```python
from build123d import *
from OCP.BRepFilletAPI import BRepFilletAPI_MakeChamfer

# Parameters (mm, degrees)
SKETCH1_W           = 16
SKETCH1_H           = 16
BOSS_EXTRUDE1_DEPTH = 10
SKETCH2_R           = 4
CUT_EXTRUDE1_DEPTH  = 1
FILLET4_SIZE        = 2
FILLET4_SIZE2       = 1.2


with BuildPart() as part:
    # Sketch1 → Boss-Extrude1 (new body)
    with BuildSketch(Plane.XY):
        with Locations((8, 8)):
            Rectangle(SKETCH1_W, SKETCH1_H)
    extrude(amount=BOSS_EXTRUDE1_DEPTH)

    # Sketch2 → Cut-Extrude1 (cut)
    with BuildSketch(Plane.XY.offset(10)):
        with Locations((8, 8)):
            Circle(SKETCH2_R)
    extrude(amount=-CUT_EXTRUDE1_DEPTH, mode=Mode.SUBTRACT)

    # Fillet4: one chamfer whose edges measure the first distance from different faces: ONE call of the kernel's chamfer builder (chamfer() names one face for all edges)
    fillet4_edges_1 = [part.edges().sort_by_distance(p)[0] for p in [
        (16, 8, 10),
    ]]
    fillet4_side_1 = [part.faces().sort_by_distance(p)[0] for p in [
        (16, 8, 5),
    ]]
    fillet4_edges_2 = [part.edges().sort_by_distance(p)[0] for p in [
        (8, 16, 10),
    ]]
    fillet4_side_2 = [part.faces().sort_by_distance(p)[0] for p in [
        (8, 16, 5),
    ]]
    fillet4_edges_3 = [part.edges().sort_by_distance(p)[0] for p in [
        (0, 8, 10),
    ]]
    fillet4_side_3 = [part.faces().sort_by_distance(p)[0] for p in [
        (0, 8, 5),
    ]]
    fillet4_edges_4 = [part.edges().sort_by_distance(p)[0] for p in [
        (8, 0, 10),
    ]]
    fillet4_side_4 = [part.faces().sort_by_distance(p)[0] for p in [
        (8, 0, 5),
    ]]
    fillet4 = BRepFilletAPI_MakeChamfer(part.part.solid().wrapped)
    for e in fillet4_edges_1:
        fillet4.Add(FILLET4_SIZE, FILLET4_SIZE2, e.wrapped, fillet4_side_1[0].wrapped)  # the first distance lies on this face
    for e in fillet4_edges_2:
        fillet4.Add(FILLET4_SIZE, FILLET4_SIZE2, e.wrapped, fillet4_side_2[0].wrapped)  # the first distance lies on this face
    for e in fillet4_edges_3:
        fillet4.Add(FILLET4_SIZE, FILLET4_SIZE2, e.wrapped, fillet4_side_3[0].wrapped)  # the first distance lies on this face
    for e in fillet4_edges_4:
        fillet4.Add(FILLET4_SIZE, FILLET4_SIZE2, e.wrapped, fillet4_side_4[0].wrapped)  # the first distance lies on this face
    add(Compound.cast(fillet4.Shape()), mode=Mode.REPLACE)


solid = part.part
```
Can you work these out from the model? Positions are in its coordinate system, mm. A direction names the side the tool comes from. Coordinates: 2 decimals unless noted, no trailing zeros. Loops run counter-clockwise (first coordinate to the right, second up) from the corner with the lowest first, then second, coordinate; pieces in that order, holes last.
Item 1: Suppose I cut it at D-D (z = 8.75). Please give me the cut outline in (x, y).
Answers below:
outline: (0.45, 0.45) - (15.55, 0.45) - (15.55, 15.55) - (0.45, 15.55) - close
Item 2: Suppose I cut it at B-B (y = 14.25). Please give me the cut outline in (x, z).
Answers below:
outline: (0, 0) - (16, 0) - (16, 8) - (14.8, 10) - (1.2, 10) - (0, 8) - close
Item 3: Suppose I cut it at A-A (x = 8). Please give me the cut outline in (y, z), then the cut area to 3 significant figures.
Answers below:
outline: (0, 0) - (16, 0) - (16, 8) - (14.8, 10) - (12, 10) - (12, 9) - (4, 9) - (4, 10) - (1.2, 10) - (0, 8) - close
area: 150 mm2
Item 4: Which directions (+Z, -Z, +X, -X, +Y, -Y) give clear straight access to the entire face, cutting with the end or side of a thin tool? Please do faces 5 (the face through (4.8, 5.6, 9.5)), 6 (the face through (0, 8, 4)).
Answers below:
face 5: +Z
face 6: +Z, -Z, -X, +Y, -Y
Item 5: If we mould it in two halves opening along X, with no side actions, what happens to faces 1 (the face through (8, 8, 9)), 2 (the face through (0.6, 7.9, 9)), 3 (the face through (7.9, 15.4, 9)), 4 (the face through (15.4, 7.9, 9))? For each: released by +X, released by -X, zero draft, split by the parting line, or undercut.
Answers below:
face 1: undercut
face 2: released by -X
face 3: zero draft
face 4: released by +X
Item 6: I'm going to push a flat-ended pin straight in: pin 1 (6.5 mm diameter, centred on x = 6, y = 6, fed in from +Z). Where does the tip first touch, or does it pass through?
Answers below:
pin 1: stops at z = 10
Item 7: Please list where these lines run through material, in increasing order: L1, parallel to Z at x = 6, y = 10.5; L2, parallel to Y at x = 8, z = 9.65; L3, parallel to Y at x = 8, z = 9.4.
Answers below:
L1: z = 0 to 9
L2: y = 0.99 to 4, 12 to 15.01
L3: y = 0.84 to 4, 12 to 15.16
